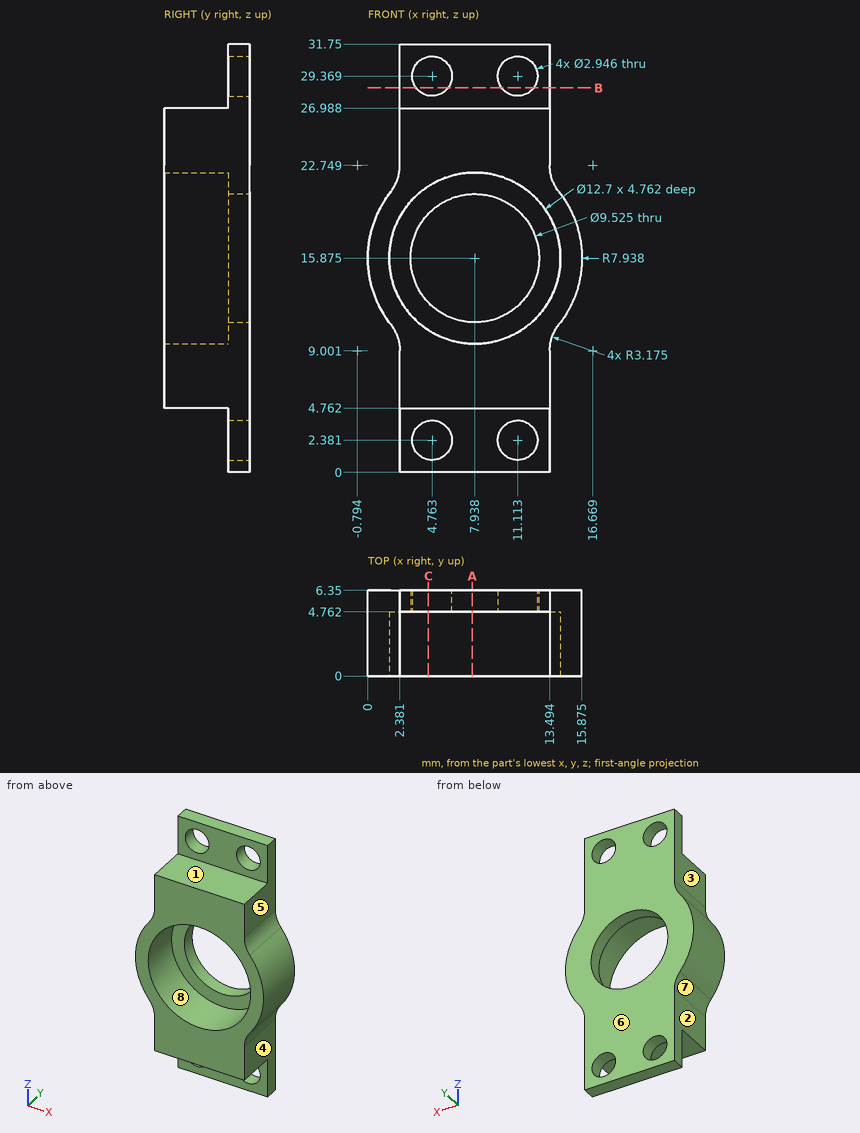
Print and shaded views of the part. All mm, measured from the part's lowest x, y and z. A direction names the side the tool comes from. Round coordinates to 2 decimals unless told otherwise and drop trailing zeros. Write each loop counter-clockwise with the first axis right and the second up, starting at its lowest first coordinate (ties: lowest second). Pieces come first, ordered by that corner, then holes. Notation, with made-up numbers: (20.25, -32.75) -> (67.25, -32.75) arc R19 cw to (67.25, -20.75) -> close; hole circle Ø10 at (-40, -37.5). An arc over 180 degrees is marked (long way). Write item = value, one per line.
(1) Probe L1, parallel to Z at x = 4.5, y = 5.5; L2, parallel to Y at x = 3, z = 13.5; L3, parallel to X at y = 0.75, z = 6. List the from-to ranges inside material, lowest first.
Answer:
L1 = 0 to 0.93, 3.83 to 12.58, 19.17 to 27.92, 30.82 to 31.75
L2 = 4.76 to 6.35
L3 = 2.38 to 13.49
(2) Tool access for the marked faces 1, 2, 3 and 4: list every direction of +Z, -Z, +X, -X, +Y, -Y with a clear straight run to the whole face (end or side of a thin tool).
Answer:
face_1 = +Z, +X, -X, -Y
face_2 = -Z, -X, +Y, -Y
face_3 = +Z, -X, +Y, -Y
face_4 = -Z, +X, +Y, -Y
(3) Two-plate mould, pull along X, no slides. Class the marked faces 5, 6, 7 and 8: pulls with the +X half, pulls with the -X half, needs draft (parallel to the pull), parting line crosses it, or undercut.
Answer:
face_5 = pulls with the +X half
face_6 = needs draft
face_7 = pulls with the -X half
face_8 = undercut
(4) Band-saw the part on C-C (x = 4.5). State how many separate pieces and enclosed holes the cut face has.
Answer:
separate_pieces = 4
enclosed_holes = 0
(5) Band-saw the part on A-A (x = 7.75). Give the cut face in (y, z).
Answer:
outline = (0, 4.76) -> (4.76, 4.76) -> (4.76, 0) -> (6.35, 0) -> (6.35, 11.12) -> (4.76, 11.12) -> (4.76, 9.53) -> (0, 9.53) -> close; (0, 22.22) -> (4.76, 22.22) -> (4.76, 20.63) -> (6.35, 20.63) -> (6.35, 31.75) -> (4.76, 31.75) -> (4.76, 26.99) -> (0, 26.99) -> close
(6) Flat gauge pins, fed straight in: pin 1 (3 mm diameter, centred on y = 4.5, z = 25.5, fed in from +X); pin 2 (3 mm diameter, centred on x = 2.5, y = 1.5, fed in from +Z); pin 3 (1.4 mm diameter, centred on x = 8, z = 2, fed in from -Y). Where does each tip first touch, or does it go through?
Answer:
pin_1 = 13.49
pin_2 = 26.99
pin_3 = 4.76
(7) Band-saw the part on B-B (z = 28.5). Give the cut face in (x, y).
Answer:
outline = (2.38, 4.76) -> (3.57, 4.76) -> (3.57, 6.35) -> (2.38, 6.35) -> close; (5.95, 4.76) -> (9.92, 4.76) -> (9.92, 6.35) -> (5.95, 6.35) -> close; (12.3, 4.76) -> (13.49, 4.76) -> (13.49, 6.35) -> (12.3, 6.35) -> close
